```python
from build123d import *

# Parameters (mm, degrees)
BOSS_EXTRUDE1_DEPTH = 18
BOSS_EXTRUDE2_REACH = 30.6
SKETCH2_R           = 4.9
BOSS_EXTRUDE3_START = 29
SKETCH3_R           = 4.9
BOSS_EXTRUDE3_DEPTH = 29
SKETCH4_R           = 1.75
CUT_EXTRUDE1_DEPTH  = 29
SKETCH5_W           = 40.000265569
SKETCH5_H           = 1.6
CUT_EXTRUDE2_DEPTH  = 40
FILLET1_R           = 5


with BuildPart() as part:
    # Sketch1 → Boss-Extrude1 (new body)
    with BuildSketch(Plane(origin=(0, 0, 0), x_dir=(1, 0, 0), z_dir=(0, 1, 0))):
        with BuildLine():
            Line((8.3059154, -19.120265102), (10.102040816, -20))
            add(Edge.make_bspline(
                [(10.101910741, 20.000265569), (13.36730358, 13.333510379), (16.63267474, 8.8523e-05), (13.367346939, -13.333333333), (10.102040816, -20)],
                knots=[0.21428192, 0.21428192, 0.21428192, 0.21428192, 0.5, 0.785714286, 0.785714286, 0.785714286, 0.785714286], degree=3))
            Line((10.101910741, 20.000265569), (8.30578994, 19.12052125))
            add(Edge.make_bspline(
                [(8.30578994, 19.12052125), (8.694326407, 18.327269829), (9.438931208, 16.706587132), (10.709549512, 13.511731918), (11.931546391, 9.520297592), (12.805878251, 4.755507519), (13.097053142, 0.000126231), (12.80590918, -4.755254756), (11.931608442, -9.520044011), (10.709637835, -13.511477312), (9.43904063, -16.706331706), (8.694446639, -18.327013824), (8.3059154, -19.120265102)],
                knots=[0.21428192, 0.21428192, 0.21428192, 0.21428192, 0.249996443, 0.285710966, 0.357140012, 0.428569057, 0.499998103, 0.571427149, 0.642856194, 0.71428524, 0.749999763, 0.785714286, 0.785714286, 0.785714286, 0.785714286], degree=3))
        make_face()
    extrude(amount=BOSS_EXTRUDE1_DEPTH)

    # Sketch2 → Boss-Extrude2 (add, up to next)
    with BuildSketch(Plane(origin=(18, 0, 0), x_dir=(0, 0, -1), z_dir=(1, 0, 0)), mode=Mode.PRIVATE) as boss_extrude2_sk1:
        with Locations((0, 9)):
            Circle(SKETCH2_R)
    boss_extrude2_tool1 = extrude(boss_extrude2_sk1.sketch, amount=-BOSS_EXTRUDE2_REACH, mode=Mode.PRIVATE) - part.part
    add(boss_extrude2_tool1.solids().sort_by_distance((18, 9, 0))[0])

    # Sketch3 → Boss-Extrude3 (add)
    with BuildSketch(Plane(origin=(18, 0, 0), x_dir=(0, 0, -1), z_dir=(1, 0, 0)).offset(BOSS_EXTRUDE3_START)):
        with Locations((0, 9)):
            Circle(SKETCH3_R)
    extrude(amount=-BOSS_EXTRUDE3_DEPTH)

    # Sketch4 → Cut-Extrude1 (cut)
    with BuildSketch(Plane(origin=(47, 0, 0), x_dir=(0, 0, -1), z_dir=(1, 0, 0))):
        with Locations((0, 9)):
            Circle(SKETCH4_R)
    extrude(amount=-CUT_EXTRUDE1_DEPTH, mode=Mode.SUBTRACT)

    # Sketch5 → Cut-Extrude2 (cut)
    with BuildSketch(Plane(origin=(47, 0, 0), x_dir=(0, 0, -1), z_dir=(1, 0, 0))):
        with Locations((0.000132784, 0.8)):
            Rectangle(SKETCH5_W, SKETCH5_H)
    extrude(amount=-CUT_EXTRUDE2_DEPTH, mode=Mode.SUBTRACT)

    # Fillet1
    # the kernel refuses this fillet: 5 mm, written as the material it takes off along each edge
    with BuildSketch(Plane(origin=(8.30578994, -7.764782929, -19.12052125), x_dir=(0.4075991497748225, 0, 0.9131609568432292), z_dir=(0, 1, 0))) as fillet1_piece_1:
        with BuildLine():
            CenterArc((3.930348167, 4.996597215), FILLET1_R, 216.83934776, 51.046703295)
            Line((-0.071250852, 1.998730426), (-0.151282833, 1.93877309))
            ThreePointArc((-0.151282833, 1.93877309), (-0.135561948, 0.99580267), (-0.099936521, -0.003562543))
            Line((-0.099936521, -0.003562543), (0.003562543, -0.099936521))
            ThreePointArc((0.003562543, -0.099936521), (1.872980998, -0.066213211), (3.742224472, -0.099931944))
            Line((3.742224472, -0.099931944), (3.745913172, 0))
        make_face()
    extrude(amount=35.129565858, mode=Mode.SUBTRACT)
    with BuildSketch(Plane(origin=(8.3059154, -7.764778421, 19.120265102), x_dir=(0.8980627079890215, 0, 0.4398674488063712), z_dir=(0, 1, 0))) as fillet1_piece_2:
        with BuildLine():
            CenterArc((4.853404013, 4.105859902), FILLET1_R, 184.155597401, 51.046688752)
            Line((-0.133450663, 3.743533478), (-0.233187757, 3.736286949))
            ThreePointArc((-0.233187757, 3.736286949), (-0.132897152, 1.869432253), (-0.1, 0))
            Line((-0.1, 0), (0, -0.1))
            ThreePointArc((0, -0.1), (1, -0.1), (1.94293192, -0.082117198))
            Line((1.94293192, -0.082117198), (2, 0))
        make_face()
    extrude(amount=35.129556842, mode=Mode.SUBTRACT)


solid = part.part
```
Verification items for the finished model (mm, model axes). A direction names the side the tool comes from. Coordinates: 2 decimals unless noted, no trailing zeros. Loops run counter-clockwise (first coordinate to the right, second up) from the corner with the lowest first, then second, coordinate; pieces in that order, holes last. Notation, with made-up numbers: (10, -24) - (14, -24) arc R23 ccw to (14, -4) - close; hole circle Ø4 at (77, 68). An arc over 180 degrees is marked (long way). Return JSON: item names as keys, results as strings.
1. Tool access check on faces 1 (the flat face through (14, 1.6, 0)), 2 (the cylindrical face through (32.703, 10.735, 0.228)). Record the directions out of +Z, -Z, +X, -X, +Y, -Y that give a thin tool (end or side, any length) a straight path to the whole face; none if there is none.
Established:
{"face 1": "+Z, -Z, +X, -X, -Y", "face 2": "+X"}
2. Thickness scan on L1, parallel to Y at x = 30, z = 0; L2, parallel to Z at x = 30.5, y = 9.5; L3, parallel to X at y = 9, z = -11. Record the ranges inside material, lowest first.
Established:
{"L1": "y = 4.1 to 7.25, 10.75 to 13.9", "L2": "z = -4.87 to -1.68, 1.68 to 4.87", "L3": "x = 11.44 to 13.52"}
3. Go/stop test with flat-tipped pins: pin 1 (8 mm diameter, centred on x = 33, y = 14, fed in from +Z); pin 2 (8 mm diameter, centred on x = 24.5, y = 9.5, fed in from +Z); pin 3 (4 mm diameter, centred on y = 7.5, z = -7, fed in from +X). Record where each tip stops, or that it passes through.
Established:
{"pin 1": "stops at z = 4.8", "pin 2": "stops at z = 4.9", "pin 3": "stops at x = 14.69"}
4. Mould release check, pull along Z, two halves, no side actions. Record for faces 3 (the cylindrical face through (9.482, 9.685, -17.912)), 4 (the cylindrical face through (31.079, 12.312, 3.612)), 5 (the flat face through (13.3, 18, -0.1)): +Z half, -Z half, draft (parallel to the pull), parting line (faces both ways), or undercut.
Established:
{"face 3": "undercut", "face 4": "parting line", "face 5": "draft"}
5. Section check A-A, the plane x = 43.5. Record the boundary of the cut face in (y, z), then the cut area to 3 significant figures.
Established:
{"outline": "circle Ø9.8 at (9, 0); hole circle Ø3.5 at (9, 0)", "area": "65.8 mm2"}
